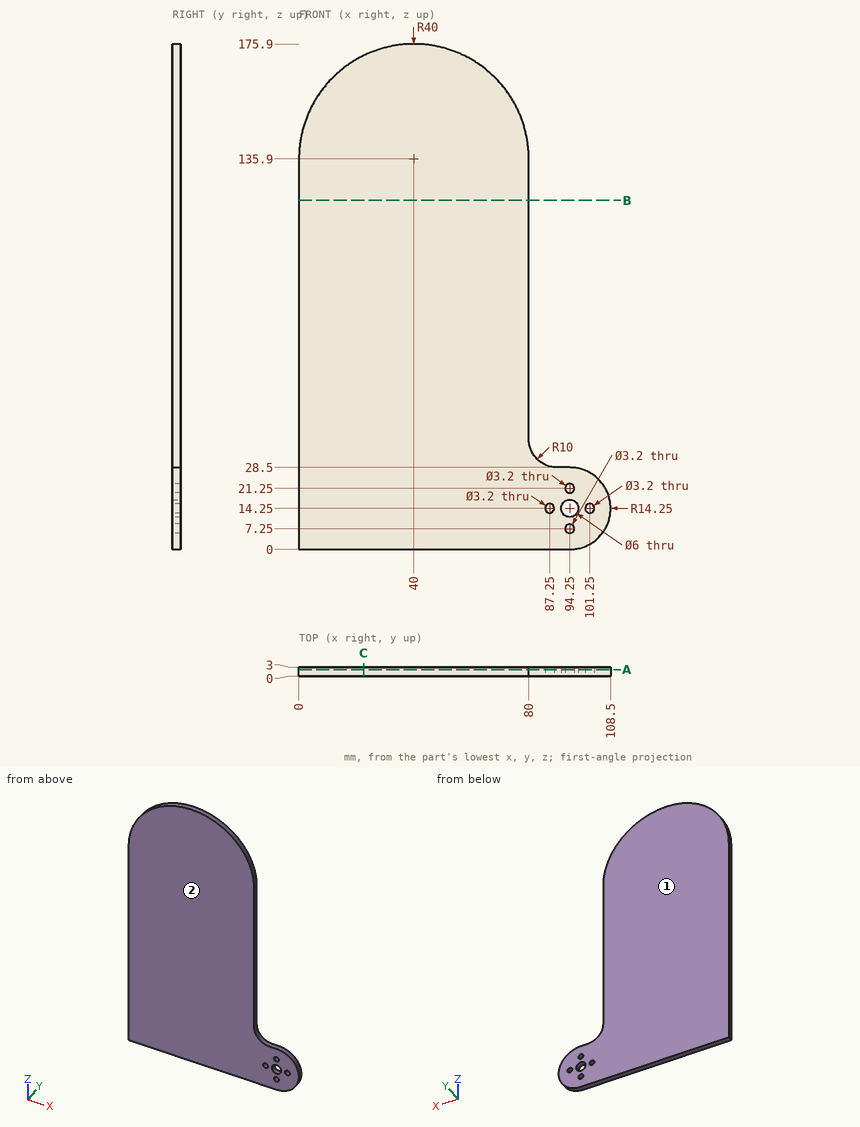
Check sheet for the drawn part. Datum: minimum x, y, z corner. Units: mm. Coordinates: 2 decimals unless noted, no trailing zeros. Write each loop counter-clockwise with the first axis right and the second up, starting at its lowest first coordinate (ties: lowest second). Pieces come first, ordered by that corner, then holes. Notation, with made-up numbers: M 15.5,15.5 L 32.5,15.5 A20 cw 32.5,39.5 Z; hole C -34.75,11.25 d11. An arc over 180 degrees is marked long. One line per item, written item: value.
Item 1: Section check A-A, the plane y = 2.25. Record the boundary of the cut face in (x, z), plus the area to 3 significant figures.
Check sheet entries:
outline: M 0,0 L 94.25,0 A14.25 ccw 94.25,28.5 L 90,28.5 A10 cw 80,38.5 L 80,135.9 A40 ccw 0,135.9 Z; hole C 87.25,14.25 d3.2; hole C 94.25,14.25 d6; hole C 94.25,7.25 d3.2; hole C 94.25,21.25 d3.2; hole C 101.25,14.25 d3.2
area: 14,100 mm^2
Item 2: Mould release check, pull along Y, two halves, no side actions. Record for the marked faces 1 and 2: pulls with the +Y half, pulls with the -Y half, needs draft (parallel to the pull), parting line crosses it, or undercut.
Check sheet entries:
face 1: pulls with the +Y half
face 2: pulls with the -Y half
Item 3: Section check C-C, the plane x = 22.5. Record the boundary of the cut face in (y, z).
Check sheet entries:
outline: M 0,0 L 3,0 L 3,171.87 L 0,171.87 Z
Item 4: Scan lines: line 1 along X through (y, z) = (0.6, 14.25); line 2 along X through (y, z) = (2.55, 126); line 3 along Z through (x, y) = (87.25, 1.45). Record each from-to range of solid material in increasing order.
Check sheet entries:
line 1: x = 0 to 85.65, 88.85 to 91.25, 97.25 to 99.65, 102.85 to 108.5
line 2: x = 0 to 80
line 3: z = 0 to 12.65, 15.85 to 28.89
Item 5: Gauge pin test, flat ends, axial feed: pin 1 Ø0.9 at (y, z) = (1.5, 106.5) entering from +X; pin 2 Ø1.5 at (x, y) = (57, 0.5) entering from +Z; pin 3 Ø5.5 at (x, z) = (94.25, 14.25) entering from -Y; pin 4 Ø0.9 at (x, y) = (92, 1.5) entering from +Z. Record the tip position at first contact, or that the pin passes through.
Check sheet entries:
pin 1: stops at x = 80
pin 2: stops at z = 172.45
pin 3: passes through
pin 4: stops at z = 28.5
Item 6: Section check B-B, the plane z = 121.5. Record the boundary of the cut face in (x, y), plus the area to 3 significant figures.
Check sheet entries:
outline: M 0,0 L 80,0 L 80,3 L 0,3 Z
area: 240 mm^2
